CAD build for the part. Positions are in the model's coordinates, mm. A direction names the side the tool comes from. Give positions to 0.01 mm unless a question says otherwise; leave off trailing zeros. Write each loop counter-clockwise with the first axis right and the second up, starting at its lowest first coordinate (ties: lowest second). Pieces come first, ordered by that corner, then holes. Notation, with made-up numbers: (-39, 74) - (-6, 74) arc R33 ccw to (-6, 105) - close; hole circle Ø6 at (37, 58). An arc over 180 degrees is marked (long way). Write item = value, one per line. Start each with the question number.
```python
from build123d import *

# Parameters (mm, degrees)
CROQUIS1_W              = 84
CROQUIS1_H              = 84
CROQUIS1_R              = 39
CROQUIS1_R_2            = 2.5
SALIENTE_EXTRUIR1_DEPTH = 1.5
REVOLUCI_N2_ANGLE       = 180
SALIENTE_EXTRUIR2_DEPTH = 20
SALIENTE_EXTRUIR3_DEPTH = 15
CROQUIS8_W              = 10.9
CROQUIS8_H              = 17.5
CROQUIS8_R              = 3.6
SALIENTE_EXTRUIR4_DEPTH = 2
SALIENTE_EXTRUIR5_DEPTH = 16.5
CROQUIS10_W             = 16.5
CROQUIS10_H             = 16.5
CROQUIS10_R             = 6.45
SALIENTE_EXTRUIR6_DEPTH = 10


with BuildPart() as part:
    # Croquis1 → Saliente-Extruir1 (new body)
    with BuildSketch(Plane.XY):
        with Locations((-61.319838057, -7.506072874)):
            Rectangle(CROQUIS1_W, CROQUIS1_H)
        with Locations((-61.319838057, -7.506072874)):
            Circle(CROQUIS1_R, mode=Mode.SUBTRACT)
        with Locations((-97.028730507, 28.202819575)):
            Circle(CROQUIS1_R_2, mode=Mode.SUBTRACT)
        with Locations((-25.528730507, 28.202819575)):
            Circle(CROQUIS1_R_2, mode=Mode.SUBTRACT)
        with Locations((-25.528730507, -43.297180425)):
            Circle(CROQUIS1_R_2, mode=Mode.SUBTRACT)
        with Locations((-97.028730507, -43.297180425)):
            Circle(CROQUIS1_R_2, mode=Mode.SUBTRACT)
    extrude(amount=SALIENTE_EXTRUIR1_DEPTH)

    # Croquis4 → Revolución2 (revolve)
    with BuildSketch(Plane(origin=(-61.319838057, -49.506072874, 1.5), x_dir=(0, 0, -1), z_dir=(1, 0, 0))):
        Polygon((-40, 27), (0, 3), (0, 2), (-40, 26), align=None)
    revolve(axis=Axis((-61.319838057, -7.506072874, 1.5), (0, 0, -1)), revolution_arc=REVOLUCI_N2_ANGLE)

    # Croquis6 → Saliente-Extruir2 (add)
    with BuildSketch(Plane.ZY.offset(103.319838057)):
        Polygon((0, -7.506072874), (0, -16.256072874), (1.5, -16.256072874), (1.5, 1.243927126), (0, 1.243927126), align=None)
    extrude(amount=SALIENTE_EXTRUIR2_DEPTH)

    # Croquis7 → Saliente-Extruir3 (add)
    with BuildSketch(Plane.ZY.offset(123.319838057)):
        Polygon((10.9, 1.243927126), (1.5, 1.243927126), (1.5, -0.756072874), (8.9, -0.756072874), (8.9, -14.256072874), (1.5, -14.256072874), (1.5, -16.256072874), (10.9, -16.256072874), align=None)
    extrude(amount=-SALIENTE_EXTRUIR3_DEPTH)

    # Croquis8 → Saliente-Extruir4 (add)
    with BuildSketch(Plane.ZY.offset(123.319838057)):
        with Locations((5.45, -7.506072874)):
            Rectangle(CROQUIS8_W, CROQUIS8_H)
        with Locations((5.45, -7.506072874)):
            Circle(CROQUIS8_R, mode=Mode.SUBTRACT)
    extrude(amount=SALIENTE_EXTRUIR4_DEPTH)

    # Croquis9 → Saliente-Extruir5 (add)
    with BuildSketch(Plane(origin=(-19.319838057, 0, 0), x_dir=(0, 0, -1), z_dir=(1, 0, 0))):
        Polygon((0, -7.506072874), (0, 0.743927126), (-1.5, 0.743927126), (-1.5, -15.756072874), (0, -15.756072874), align=None)
    extrude(amount=SALIENTE_EXTRUIR5_DEPTH)

    # Croquis10 → Saliente-Extruir6 (add)
    with BuildSketch(Plane.XY.offset(1.5)):
        with Locations((-11.069838057, -7.506072874)):
            Rectangle(CROQUIS10_W, CROQUIS10_H)
        with Locations((-11.069838057, -7.506072874)):
            Circle(CROQUIS10_R, mode=Mode.SUBTRACT)
    extrude(amount=SALIENTE_EXTRUIR6_DEPTH)


solid = part.part
```
1. Pin check, flat tips, straight feed: pin 1 Ø4 at (x, y) = (-73.5, -35.5) entering from -Z; pin 2 Ø4 at (x, y) = (-25.53, -43.3) entering from +Z; pin 3 Ø0.8 at (y, z) = (-38.5, 1) entering from +X; pin 4 Ø8 at (y, z) = (-9.5, 20) entering from -X. Stop position of each tip, or through.
2. Cut at A-A (z = 7.5). Give the cut face in (x, y), then the cut area to 3 significant figures.
3. Mould opens along X. For faces 4 (the flat face through (-125.32, -7.4, 1.7)), 5 (the flat face through (-11, 0.744, 6)), 6 (the flat face through (-116, -7, 8.9)) say: +X half, -X half, draft (parallel to the pull), parting line (faces both ways), or undercut.
4. Cut at D-D (z = 26). Give the cut face in (x, y), then the cut area to 3 significant figures.
5. Tool access for faces 1 (the flat face through (-11, -7, 1.5)), 2 (the flat face through (-108.32, -7.4, 9.3)), 3 (the flat face through (-117, -16.256, 5)): list every direction of +Z, -Z, +X, -X, +Y, -Y with a clear straight run to the whole face (end or side of a thin tool).
6. Cut at C-C (x = -11). Give the cut face in (y, z).
7. Cut at B-B (x = -110). Give the cut face in (y, z), then the cut area to 4 significant figures.
8. Wall check: line 1 along Y through (x, z) = (-124.25, 5.45); line 2 along Y through (x, z) = (-13.5, 5.5); line 3 along X through (y, z) = (-9.5, 7). Give the ranges that are in metal, low to high.
Output:
q1.pin_1 = 12.29
q1.pin_2 = through
q1.pin_3 = -19.32
q1.pin_4 = -92.57
q2.outline = (-125.32, -16.26) - (-108.32, -16.26) - (-108.32, -14.26) - (-123.32, -14.26) - (-123.32, -10.47) - (-125.32, -10.47) - close; (-125.32, -4.55) - (-123.32, -4.55) - (-123.32, -0.76) - (-108.32, -0.76) - (-108.32, 1.24) - (-125.32, 1.24) - close; (-61.32, -43.91) - (-61.32, -42.91) arc R35.4 cw to (-61.32, 27.89) - (-61.32, 28.89) arc R36.4 ccw to start; (-19.32, -15.76) - (-2.82, -15.76) - (-2.82, 0.74) - (-19.32, 0.74) - close; hole circle Ø12.9 at (-11.07, -7.51)
q2.area = 337 mm2
q3.face_4 = -X half
q3.face_5 = draft
q3.face_6 = undercut
q4.outline = (-61.32, -32.81) - (-61.32, -31.81) arc R24.3 cw to (-61.32, 16.79) - (-61.32, 17.79) arc R25.3 ccw to start
q4.area = 77.9 mm2
q5.face_1 = +Z
q5.face_2 = +Z, +Y, -Y
q5.face_3 = +Z, -Z, -X, -Y
q6.outline = (-15.76, 0) - (0.74, 0) - (0.74, 11.5) - (-1.06, 11.5) - (-1.06, 1.5) - (-13.96, 1.5) - (-13.96, 11.5) - (-15.76, 11.5) - close
q7.outline = (-16.26, 0) - (1.24, 0) - (1.24, 10.9) - (-16.26, 10.9) - close; hole (-14.26, 1.5) - (-0.76, 1.5) - (-0.76, 8.9) - (-14.26, 8.9) - close
q7.area = 90.85 mm2
q8.line_1 = -16.26 to -11.11, -3.91 to 1.24
q8.line_2 = -15.76 to -13.48, -1.53 to 0.74
q8.line_3 = -97.97 to -96.96, -19.32 to -17.2, -4.94 to -2.82
